```python
from build123d import *

# Parameters (mm, degrees)
SKETCH_W  = 15
SKETCH_H  = 5
PAD_DEPTH = 3


with BuildPart() as part:
    # Sketch → Pad (new body)
    with BuildSketch(Plane.XY):
        Polygon((-60.255625, 82.82953), (94.744375, 82.82953), (94.744375, -67.17047), (59.744375, -67.17047), (59.744375, -17.17047), (44.744375, -17.17047), (44.744375, -67.17047), (-10.255625, -67.17047), (-10.255625, -17.17047), (-25.255625, -17.17047), (-25.255625, -67.17047), (-60.255625, -67.17047), align=None)
        with Locations((-12.755625, 70.32953)):
            Rectangle(SKETCH_W, SKETCH_H, mode=Mode.SUBTRACT)
        with Locations((47.244375, 70.32953)):
            Rectangle(SKETCH_W, SKETCH_H, mode=Mode.SUBTRACT)
    extrude(amount=PAD_DEPTH)


solid = part.part
```
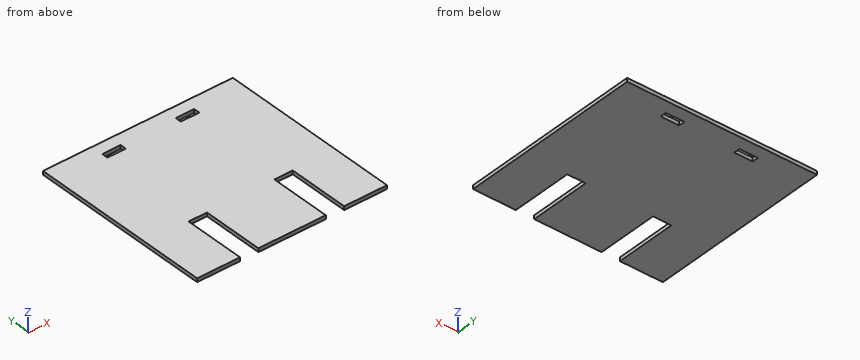
The listing builds one solid part. Answer for the finished solid, in the listing's coordinates (mm). Round coordinates to 2 decimals unless told otherwise and drop trailing zeros. Loops run counter-clockwise (first coordinate to the right, second up) from the corner with the lowest first, then second, coordinate; pieces in that order, holes last. Notation, with made-up numbers: (57.5, -4) -> (101.5, -4) arc R22 cw to (101.5, 25) -> close; hole circle Ø7 at (77.5, 2.5). An arc over 180 degrees is marked (long way). Use one line per item in the form item = value.
1. The part is cut by section B-B on x = -15.5. Determine the outline of the cut face in (y, z), and give its area (3 significant figures).
Answer key:
outline = (-17.17, 0) -> (67.83, 0) -> (67.83, 3) -> (-17.17, 3) -> close; (72.83, 0) -> (82.83, 0) -> (82.83, 3) -> (72.83, 3) -> close
area = 285 mm²
2. The part is cut by section D-D on x = 42.5. Determine the outline of the cut face in (y, z).
Answer key:
outline = (-67.17, 0) -> (67.83, 0) -> (67.83, 3) -> (-67.17, 3) -> close; (72.83, 0) -> (82.83, 0) -> (82.83, 3) -> (72.83, 3) -> close
3. The part is cut by section A-A on y = -56.5. Determine the outline of the cut face in (x, z), and give its area (3 significant figures).
Answer key:
outline = (-60.26, 0) -> (-25.26, 0) -> (-25.26, 3) -> (-60.26, 3) -> close; (-10.26, 0) -> (44.74, 0) -> (44.74, 3) -> (-10.26, 3) -> close; (59.74, 0) -> (94.74, 0) -> (94.74, 3) -> (59.74, 3) -> close
area = 375 mm²
4. A flat-ended cylindrical pin translates along its axis: pin 1 Ø1.5 at (x, z) = (55.5, 2) entering from -Y. Find the tip coordinate at first contact, or state that the pin passes through.
Answer key:
pin_1 = -17.17
5. The part is cut by section C-C on z = 1.2. Determine the outline of the cut face in (x, y), and give its area (3 significant figures).
Answer key:
outline = (-60.26, -67.17) -> (-25.26, -67.17) -> (-25.26, -17.17) -> (-10.26, -17.17) -> (-10.26, -67.17) -> (44.74, -67.17) -> (44.74, -17.17) -> (59.74, -17.17) -> (59.74, -67.17) -> (94.74, -67.17) -> (94.74, 82.83) -> (-60.26, 82.83) -> close; hole (-20.26, 67.83) -> (-5.26, 67.83) -> (-5.26, 72.83) -> (-20.26, 72.83) -> close; hole (39.74, 67.83) -> (54.74, 67.83) -> (54.74, 72.83) -> (39.74, 72.83) -> close
area = 21,600 mm²
6. Find the intervals of material crossed by probe 1 along X at (y, z) = (-28, 1.7); probe 2 along Y at (x, z) = (51, 1.05); probe 3 along Y at (x, z) = (44.5, 2.8), in increasing order. Write a range as [from, to].
Answer key:
probe_1 = [-60.26, -25.26], [-10.26, 44.74], [59.74, 94.74]
probe_2 = [-17.17, 67.83], [72.83, 82.83]
probe_3 = [-67.17, 67.83], [72.83, 82.83]
